Work out the finished part from the listing and answer in its coordinate system (mm). Give positions to 0.01 mm unless a question says otherwise; leave off trailing zeros. Write each loop counter-clockwise with the first axis right and the second up, starting at its lowest first coordinate (ties: lowest second). Pieces come first, ordered by that corner, then holes. Notation, with made-up numbers: (54, 31.25) -> (109, 31.25) arc R21 cw to (109, 40.25) -> close; hole circle Ø8 at (-40, 28). An arc over 180 degrees is marked (long way). Use a Markdown table: item, result. Add a question column.
Q1. Section A-A, the plane z = -3 is taken. Give the vertices of the cut face in (x, y), plus the area to 3 significant figures.
Q2. Consider line 1 (X direction, y = 140, z = -3.85); line 2 (X direction, y = 141, z = -4.25); line 3 (X direction, y = 41.5, z = -2). Determine where each line is inside the solid, lowest interval first.
Q3. Each of these flat-tipped pins is pushed along its axis until it touches: pin 1 Ø6 at (y, z) = (50.5, 0) entering from +X; pin 2 Ø1.5 at (x, y) = (61, 140) entering from -Z; pin 3 Ø3 at (y, z) = (33, -3) entering from +X. Where does it stop, or does it pass through?
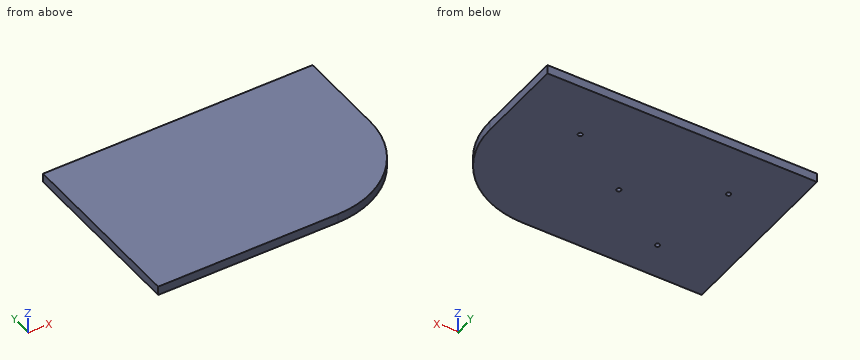
from build123d import *

# Parameters (mm, degrees)
BOSS_EXTRUDE1_DEPTH = 5
SKETCH6_R           = 2.5
CUT_EXTRUDE1_DEPTH  = 5


with BuildPart() as part:
    # Sketch1 → Boss-Extrude1 (new body, symmetric)
    with BuildSketch(Plane.XY):
        with BuildLine():
            Line((0, 200), (0, 0))
            Line((0, 0), (200, 0))
            ThreePointArc((200, 0), (270.710678119, 29.289321881), (300, 100))
            Line((300, 100), (300, 200))
            Line((300, 200), (0, 200))
        make_face()
    extrude(amount=BOSS_EXTRUDE1_DEPTH, both=True)

    # Sketch6 → Cut-Extrude1 (cut)
    with BuildSketch(Plane(origin=(0, 0, -5), x_dir=(-1, 0, 0), z_dir=(0, 0, -1))):
        with Locations((-225, 140)):
            Circle(SKETCH6_R)
        with Locations((-150, 90)):
            Circle(SKETCH6_R)
        with Locations((-60, 140)):
            Circle(SKETCH6_R)
        with Locations((-75, 40)):
            Circle(SKETCH6_R)
    extrude(amount=-CUT_EXTRUDE1_DEPTH, mode=Mode.SUBTRACT)


solid = part.part
Result set:
| question | item | result |
|---|---|---|
| 1 | outline | (0, 0) -> (200, 0) arc R100 ccw to (300, 100) -> (300, 200) -> (0, 200) -> close; hole circle Ø5 at (60, 140); hole circle Ø5 at (75, 40); hole circle Ø5 at (150, 90); hole circle Ø5 at (225, 140) |
| 1 | area | 57,800 mm2 |
| 2 | line 1 | x = 0 to 57.5, 62.5 to 222.5, 227.5 to 300 |
| 2 | line 2 | x = 0 to 57.71, 62.29 to 222.71, 227.29 to 300 |
| 2 | line 3 | x = 0 to 73, 77 to 281.1 |
| 3 | pin 1 | stops at x = 288.53 |
| 3 | pin 2 | stops at z = 0 |
| 3 | pin 3 | stops at x = 275.56 |
